Check sheet for the drawn part. Datum: minimum x, y, z corner. Units: mm. A direction names the side the tool comes from. Coordinates: 2 decimals unless noted, no trailing zeros. Order: outer loops, then holes, each group sorted by start corner. A loop starts at its lowest first (then second) coordinate and runs counter-clockwise, first axis right, second up. Notation, with made-up numbers: M -29.75,69 L 23.25,69 A31 ccw 23.25,108 Z; hole C -7.5,10.25 d8. An arc over 180 degrees is marked long. Return JSON: item names as keys, results as strings. Group by question number.
Q1. Section check D-D, the plane y = 1.85. Enter the section's corners in (x, z), then the cut area to 3 significant figures.
Q2. Section check B-B, the plane x = 6. Enter the section's corners in (y, z).
Q3. Access from +Z, -Z, +X, -X, +Y, -Y to the whole of each face (thin tool, end or side, straight path). Record for the marked faces 4 and 5.
Q4. Section check C-C, the plane y = 3.75. Enter the section's corners in (x, z).
Q5. Section check A-A, the plane z = 4. Enter the section's corners in (x, y).
Q6. Thickness scan on probe 1 along X at (y, z) = (2.1, 5); probe 2 along X at (y, z) = (3.25, 4); probe 3 along Y at (x, z) = (11.5, 6.5). Record the ranges inside material, lowest first.
Q7. Mould release check, pull along X, two halves, no side actions. Record for the marked faces 1, 2 and 3: pulls with the +X half, pulls with the -X half, needs draft (parallel to the pull), parting line crosses it, or undercut.
Q8. Go/stop test with flat-tipped pins: pin 1 Ø2.5 at (x, z) = (12.5, 1) entering from +Y; pin 2 Ø0.8 at (x, y) = (1.5, 3.5) entering from +Z. Record where each tip stops, or that it passes through.
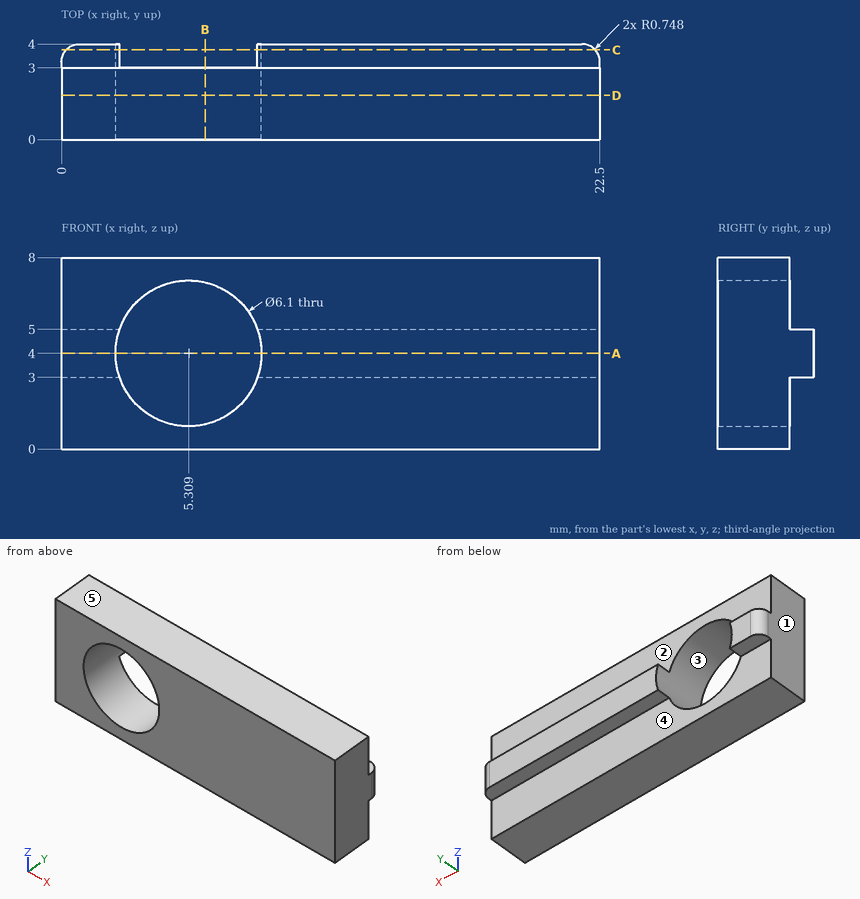
Numbers:
{
 "1": {"outline": "M 0,0 L 22.5,0 L 22.5,8 L 0,8 Z; hole C 5.31,4 d6.1", "area": "151 mm2"},
 "2": {"outline": "M 0,0 L 3,0 L 3,1.03 L 0,1.03 Z; M 0,6.97 L 3,6.97 L 3,8 L 0,8 Z"},
 "3": {"face 4": "-Z, +X, -X, +Y", "face 5": "+Z, +X, -X, +Y, -Y"},
 "4": {"outline": "M 0.19,3 L 2.43,3 A3.05 cw 2.43,5 L 0.19,5 Z; M 8.19,3 L 22.31,3 L 22.31,5 L 8.19,5 A3.05 cw Z"},
 "5": {"outline": "M 0,0 L 2.26,0 L 2.26,4 L 0.75,4 A0.75 ccw 0,3.25 Z; M 8.36,0 L 22.5,0 L 22.5,3.25 A0.75 ccw 21.75,4 L 8.36,4 Z"},
 "6": {"probe 1": "x = 0 to 2.43, 8.19 to 22.5", "probe 2": "x = 0 to 2.26, 8.36 to 22.5", "probe 3": "y = 0 to 3"},
 "7": {"face 1": "pulls with the -X half", "face 2": "needs draft", "face 3": "undercut"},
 "8": {"pin 1": "stops at y = 3", "pin 2": "stops at z = 5"}
}
